Here's how the part is built. I have some questions about the finished solid (model axes, mm). A direction names the side the tool comes from. Round coordinates to 2 decimals unless told otherwise and drop trailing zeros. Write each loop counter-clockwise with the first axis right and the second up, starting at its lowest first coordinate (ties: lowest second). Pieces come first, ordered by that corner, then holes. Notation, with made-up numbers: (-19, -10) - (6, -10) arc R8 ccw to (6, -2) - close; hole circle Ø11 at (56, 67). An arc over 180 degrees is marked (long way). Write item = value, one per line. Start each with the question number.
Item 1: If we section it at A-A (x = -2): Please give me the cut outline in (y, z), and give its area (3 significant figures).
Item 2: Thinking about a two-plate mould opening in Y: for faces 1 (the face through (-44.2, 0, 1)), 2 (the face through (46, 20, 6)), 3 (the face through (-1, -22.1, 1)), which applies, pulls with the +Y half, pulls with the -Y half, needs draft (parallel to the pull), parting line crosses it, or undercut?
Item 3: For P1, Ø2.5, axis at x = 45.5, y = 21, coming from the +Z side, with a flat end and sliding along its axis, tell me the tip position at first contact or that it passes through.
Item 4: If we section it at D-D (x = 46.3): Please give me the cut outline in (y, z).
Item 5: If I drill on line 1 along Y through (x, z) = (-33, 0.35); line 2 along X through (y, z) = (-4, 1.4); line 3 along X through (y, z) = (-19, 3.15), over which ranges is the centre line in solid material (lowest first)? Write a range as [from, to].
Item 6: If we section it at B-B (y = -5): Please give me the cut outline in (x, z).
Item 7: Which directions (+Z, -Z, +X, -X, +Y, -Y) give clear straight access to the entire face, cutting with the end or side of a thin tool? Please do faces 4 (the face through (-47.41, 21.21, 2.99)), 5 (the face through (-2, 20, 6)).
Item 8: If we section it at C-C (y = 20.2): Please give me the cut outline in (x, z), and give its area (3 significant figures).
```python
from build123d import *

# Parameters (mm, degrees)
SKETCH1_W           = 96.4
SKETCH1_H           = 44.2
SKETCH1_W_2         = 88.4
SKETCH1_H_2         = 36.2
BOSS_EXTRUDE1_DEPTH = 2
SKETCH2_R           = 1
BOSS_EXTRUDE2_DEPTH = 4
SKETCH3_R           = 1.5
BOSS_EXTRUDE3_DEPTH = 2


with BuildPart() as part:
    # Sketch1 → Boss-Extrude1 (new body)
    with BuildSketch(Plane.XY):
        Rectangle(SKETCH1_W, SKETCH1_H)
        Rectangle(SKETCH1_W_2, SKETCH1_H_2, mode=Mode.SUBTRACT)
    extrude(amount=BOSS_EXTRUDE1_DEPTH)

    # Sketch2 → Boss-Extrude2 (add)
    with BuildSketch(Plane.XY.offset(2)):
        with Locations((-46.3, 20.2)):
            Circle(SKETCH2_R)
        with Locations((-46.3, -19.2)):
            Circle(SKETCH2_R)
        with Locations((46.3, -19.2)):
            Circle(SKETCH2_R)
        with Locations((46.3, 20.2)):
            Circle(SKETCH2_R)
        with Locations((-2, 20.2)):
            Circle(SKETCH2_R)
        with Locations((-2, -20.862445561)):
            Circle(SKETCH2_R)
        with Locations((2, 20.2)):
            Circle(SKETCH2_R)
        with Locations((2, -20.862445561)):
            Circle(SKETCH2_R)
    extrude(amount=BOSS_EXTRUDE2_DEPTH)

    # Sketch3 → Boss-Extrude3 (add)
    with BuildSketch(Plane.XY.offset(2)):
        with Locations((-46.3, 20.2)):
            Circle(SKETCH3_R)
        with Locations((-46.3, -19.2)):
            Circle(SKETCH3_R)
        with Locations((46.3, -19.2)):
            Circle(SKETCH3_R)
        with Locations((46.3, 20.2)):
            Circle(SKETCH3_R)
    extrude(amount=BOSS_EXTRUDE3_DEPTH)


solid = part.part
```
Reply:
q1.outline = (-22.1, 0) - (-18.1, 0) - (-18.1, 2) - (-19.86, 2) - (-19.86, 6) - (-21.86, 6) - (-21.86, 2) - (-22.1, 2) - close; (18.1, 0) - (22.1, 0) - (22.1, 2) - (21.2, 2) - (21.2, 6) - (19.2, 6) - (19.2, 2) - (18.1, 2) - close
q1.area = 32.0 mm2
q2.face_1 = undercut
q2.face_2 = needs draft
q2.face_3 = pulls with the -Y half
q3.P1 = 6
q4.outline = (-22.1, 0) - (22.1, 0) - (22.1, 2) - (21.7, 2) - (21.7, 4) - (21.2, 4) - (21.2, 6) - (19.2, 6) - (19.2, 4) - (18.7, 4) - (18.7, 2) - (-17.7, 2) - (-17.7, 4) - (-18.2, 4) - (-18.2, 6) - (-20.2, 6) - (-20.2, 4) - (-20.7, 4) - (-20.7, 2) - (-22.1, 2) - close
q5.line_1 = [-22.1, -18.1], [18.1, 22.1]
q5.line_2 = [-48.2, -44.2], [44.2, 48.2]
q5.line_3 = [-47.79, -44.81], [44.81, 47.79]
q6.outline = (-48.2, 0) - (-44.2, 0) - (-44.2, 2) - (-48.2, 2) - close; (44.2, 0) - (48.2, 0) - (48.2, 2) - (44.2, 2) - close
q7.face_4 = +Z
q7.face_5 = +Z, +X, -X, +Y, -Y
q8.outline = (-48.2, 0) - (48.2, 0) - (48.2, 2) - (47.8, 2) - (47.8, 4) - (47.3, 4) - (47.3, 6) - (45.3, 6) - (45.3, 4) - (44.8, 4) - (44.8, 2) - (3, 2) - (3, 6) - (1, 6) - (1, 2) - (-1, 2) - (-1, 6) - (-3, 6) - (-3, 2) - (-44.8, 2) - (-44.8, 4) - (-45.3, 4) - (-45.3, 6) - (-47.3, 6) - (-47.3, 4) - (-47.8, 4) - (-47.8, 2) - (-48.2, 2) - close
q8.area = 229 mm2
